from build123d import *

# Parameters (mm, degrees)
F2_SIZE      = 1
F4_DEPTH     = 0.5
F5_T4_DEPTH  = 4.9533840607
F5_T10_DEPTH = 4.9533840607
F5_T16_DEPTH = 4.9533840607
F5_T22_DEPTH = 4.9533840607
F7_DEPTH     = 0.5
F8_T4_DEPTH  = 4.9533840607
F8_T10_DEPTH = 4.9533840607
F8_T16_DEPTH = 4.9533840607
F8_T22_DEPTH = 4.9533840607
F8_T28_DEPTH = 4.9533840607
F8_T34_DEPTH = 4.9533840607
F8_T40_DEPTH = 4.9533840607
F8_T46_DEPTH = 4.9533840607


# Not quite as in the source:
# - a fillet or chamfer that OpenCascade refuses, or shapes differently, is made with other operations: its cross-section is extruded or revolved along the edge and cut away or added


with BuildPart() as f1:
    # F0 (on Right) → F1 (revolve)
    with BuildSketch(Plane.YZ):
        with BuildLine():
            Line((0, 2), (0, 0))
            Line((0, 0), (11, 0))
            Line((11, 0), (11, 1))
            Line((11, 1), (1.5, 1))
            Line((1.5, 1), (1.5, 2.5))
            ThreePointArc((1.5, 2.5), (1.3535533906, 2.8535533906), (1, 3))
            ThreePointArc((1, 3), (0.2928932188, 2.7071067812), (0, 2))
        make_face()
    revolve(axis=Axis((0, -4.3078260496, 0), (0, -1, 0)))

    # F2
    f2_edges = [f1.edges().sort_by_distance(p)[0] for p in [
        (0, 11, -1),
    ]]
    chamfer(f2_edges, length=F2_SIZE)

    # F3 (on Right) → F4 (cut, symmetric)
    with BuildSketch(Plane.YZ):
        Polygon((1.5, 0), (0, 1.85), (0, -1.85), align=None)
    extrude(amount=F4_DEPTH, both=True, mode=Mode.SUBTRACT)

    # F5: chamfer of 0.5 on 4 edges, made by hand


with BuildPart() as f5_tool2:
    # F5_s3 → F5_t4 (new body)
    with BuildSketch(Plane(origin=(0, -1.7148497309, -2.1149813348), x_dir=(1, 0, 0), z_dir=(0, 0.6298019584, 0.7767557487))):
        Polygon((0, 1.1651336231), (0.5, 0.6651336231), (0.5, 1.1651336231), align=None)
    extrude(amount=F5_T4_DEPTH)

    split(bisect_by=Plane.XZ, keep=Keep.BOTTOM)

    split(bisect_by=Plane(origin=(0, 0.9050242398, 0.7338034376), x_dir=(1, 0, 0), z_dir=(0, -0.7767557487, -0.6298019584)), keep=Keep.TOP)


with BuildPart() as f1_1:
    add(f1.part)

    # F5_t1: union F5_tool2
    add(f5_tool2.part)


with BuildPart() as f5_tool8:
    # F5_s9 → F5_t10 (new body)
    with BuildSketch(Plane(origin=(0, -1.7148497309, -2.1149813348), x_dir=(1, 0, 0), z_dir=(0, 0.6298019584, 0.7767557487))):
        Polygon((-0.5, 0.6651336231), (0, 1.1651336231), (-0.5, 1.1651336231), align=None)
    extrude(amount=F5_T10_DEPTH)

    split(bisect_by=Plane.XZ, keep=Keep.BOTTOM)

    split(bisect_by=Plane(origin=(0, 0.9050242398, 0.7338034376), x_dir=(1, 0, 0), z_dir=(0, -0.7767557487, -0.6298019584)), keep=Keep.TOP)


with BuildPart() as f1_2:
    add(f1_1.part)

    # F5_t7: union F5_tool8
    add(f5_tool8.part)


with BuildPart() as f5_tool14:
    # F5_s15 → F5_t16 (new body)
    with BuildSketch(Plane(origin=(0, 1.4048012514, -1.73258821), x_dir=(1, 0, 0), z_dir=(0, -0.6298019584, 0.7767557487))):
        Polygon((-0.5, 0.6651336231), (0, 1.1651336231), (-0.5, 1.1651336231), align=None)
    extrude(amount=F5_T16_DEPTH)

    split(bisect_by=Plane.XZ, keep=Keep.BOTTOM)

    split(bisect_by=Plane(origin=(0, 0.9050242398, -0.7338034376), x_dir=(1, 0, 0), z_dir=(0, -0.7767557487, 0.6298019584)), keep=Keep.TOP)


with BuildPart() as f1_3:
    add(f1_2.part)

    # F5_t13: union F5_tool14
    add(f5_tool14.part)


with BuildPart() as f5_tool20:
    # F5_s21 → F5_t22 (new body)
    with BuildSketch(Plane(origin=(0, 1.4048012514, -1.73258821), x_dir=(1, 0, 0), z_dir=(0, -0.6298019584, 0.7767557487))):
        Polygon((0.5, 0.6651336231), (0, 1.1651336231), (0.5, 1.1651336231), align=None)
    extrude(amount=F5_T22_DEPTH)

    split(bisect_by=Plane.XZ, keep=Keep.BOTTOM)

    split(bisect_by=Plane(origin=(0, 0.9050242398, -0.7338034376), x_dir=(1, 0, 0), z_dir=(0, -0.7767557487, 0.6298019584)), keep=Keep.TOP)


with BuildPart() as f1_4:
    add(f1_3.part)

    # F5_t19: union F5_tool20
    add(f5_tool20.part)

    # F6 (on Top) → F7 (cut, symmetric)
    with BuildSketch(Plane.XY):
        Polygon((0, 1.5), (-1.85, 0), (1.85, 0), align=None)
    extrude(amount=F7_DEPTH, both=True, mode=Mode.SUBTRACT)

    # F8: chamfer of 0.5 on 4 edges, made by hand


with BuildPart() as f8_tool2:
    # F8_s3 → F8_t4 (new body)
    with BuildSketch(Plane(origin=(2.1149813348, -1.7148497309, 0), x_dir=(0, 0, 1), z_dir=(-0.7767557487, 0.6298019584, 0))):
        Polygon((0, 1.1651336231), (-0.5, 0.6651336231), (-0.5, 1.1651336231), align=None)
    extrude(amount=F8_T4_DEPTH)

    split(bisect_by=Plane.XZ, keep=Keep.BOTTOM)

    split(bisect_by=Plane(origin=(0.5825668116, 0.4525121199, -0.3669017188), x_dir=(-0.6134375783, 0.7897432099, 0), z_dir=(0.7071067812, 0.5492492572, -0.4453372356)), keep=Keep.TOP)


with BuildPart() as f1_5:
    add(f1_4.part)

    # F8_t1: union F8_tool2
    add(f8_tool2.part)


with BuildPart() as f8_tool8:
    # F8_s9 → F8_t10 (new body)
    with BuildSketch(Plane(origin=(2.1149813348, -1.7148497309, 0), x_dir=(0, 0, 1), z_dir=(-0.7767557487, 0.6298019584, 0))):
        Polygon((0, 1.1651336231), (-0.5, 0.6651336231), (-0.5, 1.1651336231), align=None)
    extrude(amount=F8_T10_DEPTH)

    split(bisect_by=Plane(origin=(-0.5825668116, 0.4525121199, -0.3669017188), x_dir=(-0.6134375783, -0.7897432099, 0), z_dir=(-0.7071067812, 0.5492492572, -0.4453372356)), keep=Keep.TOP)

    split(bisect_by=Plane(origin=(-0.7338034376, 0.9050242398, 0), x_dir=(0, 0, 1), z_dir=(0.6298019584, -0.7767557487, 0)), keep=Keep.TOP)


with BuildPart() as f1_6:
    add(f1_5.part)

    # F8_t7: union F8_tool8
    add(f8_tool8.part)


with BuildPart() as f8_tool14:
    # F8_s15 → F8_t16 (new body)
    with BuildSketch(Plane(origin=(1.73258821, 1.4048012514, 0), x_dir=(0, 0, 1), z_dir=(-0.7767557487, -0.6298019584, 0))):
        Polygon((-0.5, 0.6651336231), (0, 1.1651336231), (-0.5, 1.1651336231), align=None)
    extrude(amount=F8_T16_DEPTH)

    split(bisect_by=Plane(origin=(0.7338034376, 0.9050242398, 0), x_dir=(0, 0, 1), z_dir=(-0.6298019584, -0.7767557487, 0)), keep=Keep.TOP)

    split(bisect_by=Plane(origin=(0.5825668116, 0.4525121199, -0.3669017188), x_dir=(-0.6134375783, 0.7897432099, 0), z_dir=(0.7071067812, 0.5492492572, -0.4453372356)), keep=Keep.TOP)


with BuildPart() as f1_7:
    add(f1_6.part)

    # F8_t13: union F8_tool14
    add(f8_tool14.part)


with BuildPart() as f8_tool20:
    # F8_s21 → F8_t22 (new body)
    with BuildSketch(Plane(origin=(1.73258821, 1.4048012514, 0), x_dir=(0, 0, 1), z_dir=(-0.7767557487, -0.6298019584, 0))):
        Polygon((-0.5, 0.6651336231), (0, 1.1651336231), (-0.5, 1.1651336231), align=None)
    extrude(amount=F8_T22_DEPTH)

    split(bisect_by=Plane.XZ, keep=Keep.BOTTOM)

    split(bisect_by=Plane(origin=(-0.5825668116, 0.4525121199, -0.3669017188), x_dir=(-0.6134375783, -0.7897432099, 0), z_dir=(-0.7071067812, 0.5492492572, -0.4453372356)), keep=Keep.TOP)


with BuildPart() as f1_8:
    add(f1_7.part)

    # F8_t19: union F8_tool20
    add(f8_tool20.part)


with BuildPart() as f8_tool26:
    # F8_s27 → F8_t28 (new body)
    with BuildSketch(Plane(origin=(2.1149813348, -1.7148497309, 0), x_dir=(0, 0, 1), z_dir=(-0.7767557487, 0.6298019584, 0))):
        Polygon((0, 1.1651336231), (0.5, 0.6651336231), (0.5, 1.1651336231), align=None)
    extrude(amount=F8_T28_DEPTH)

    split(bisect_by=Plane.XZ, keep=Keep.BOTTOM)

    split(bisect_by=Plane(origin=(0.5825668116, 0.4525121199, 0.3669017188), x_dir=(-0.6134375783, 0.7897432099, 0), z_dir=(0.7071067812, 0.5492492572, 0.4453372356)), keep=Keep.TOP)


with BuildPart() as f1_9:
    add(f1_8.part)

    # F8_t25: union F8_tool26
    add(f8_tool26.part)


with BuildPart() as f8_tool32:
    # F8_s33 → F8_t34 (new body)
    with BuildSketch(Plane(origin=(2.1149813348, -1.7148497309, 0), x_dir=(0, 0, 1), z_dir=(-0.7767557487, 0.6298019584, 0))):
        Polygon((0, 1.1651336231), (0.5, 0.6651336231), (0.5, 1.1651336231), align=None)
    extrude(amount=F8_T34_DEPTH)

    split(bisect_by=Plane(origin=(-0.5825668116, 0.4525121199, 0.3669017188), x_dir=(-0.6134375783, -0.7897432099, 0), z_dir=(-0.7071067812, 0.5492492572, 0.4453372356)), keep=Keep.TOP)

    split(bisect_by=Plane(origin=(-0.7338034376, 0.9050242398, 0), x_dir=(0, 0, 1), z_dir=(0.6298019584, -0.7767557487, 0)), keep=Keep.TOP)


with BuildPart() as f1_10:
    add(f1_9.part)

    # F8_t31: union F8_tool32
    add(f8_tool32.part)


with BuildPart() as f8_tool38:
    # F8_s39 → F8_t40 (new body)
    with BuildSketch(Plane(origin=(1.73258821, 1.4048012514, 0), x_dir=(0, 0, 1), z_dir=(-0.7767557487, -0.6298019584, 0))):
        Polygon((0, 1.1651336231), (0.5, 0.6651336231), (0.5, 1.1651336231), align=None)
    extrude(amount=F8_T40_DEPTH)

    split(bisect_by=Plane(origin=(0.5825668116, 0.4525121199, 0.3669017188), x_dir=(-0.6134375783, 0.7897432099, 0), z_dir=(0.7071067812, 0.5492492572, 0.4453372356)), keep=Keep.TOP)

    split(bisect_by=Plane(origin=(0.7338034376, 0.9050242398, 0), x_dir=(0, 0, 1), z_dir=(-0.6298019584, -0.7767557487, 0)), keep=Keep.TOP)


with BuildPart() as f1_11:
    add(f1_10.part)

    # F8_t37: union F8_tool38
    add(f8_tool38.part)


with BuildPart() as f8_tool44:
    # F8_s45 → F8_t46 (new body)
    with BuildSketch(Plane(origin=(1.73258821, 1.4048012514, 0), x_dir=(0, 0, 1), z_dir=(-0.7767557487, -0.6298019584, 0))):
        Polygon((0, 1.1651336231), (0.5, 0.6651336231), (0.5, 1.1651336231), align=None)
    extrude(amount=F8_T46_DEPTH)

    split(bisect_by=Plane.XZ, keep=Keep.BOTTOM)

    split(bisect_by=Plane(origin=(-0.5825668116, 0.4525121199, 0.3669017188), x_dir=(-0.6134375783, -0.7897432099, 0), z_dir=(-0.7071067812, 0.5492492572, 0.4453372356)), keep=Keep.TOP)


with BuildPart() as f1_12:
    add(f1_11.part)

    # F8_t43: union F8_tool44
    add(f8_tool44.part)


solid = f1_12.part
CAD build for the part. Positions are in the model's coordinates, mm. A direction names the side the tool comes from. Give positions to 0.01 mm unless a question says otherwise; leave off trailing zeros. Order: outer loops, then holes, each group sorted by start corner. A loop starts at its lowest first (then second) coordinate and runs counter-clockwise, first axis right, second up. Notation, with made-up numbers: (8, 48.5) - (58, 48.5) arc R26 ccw to (58, 75.5) - close; hole circle Ø6 at (-11.5, 76). An arc over 180 degrees is marked (long way). Answer in a Markdown table with one row per item.
1. Saw through at A-A, the plane y = 4.75. Give the cut face in (x, z).
Data:
| item | result |
|---|---|
| outline | circle Ø2 at (0, 0) |
2. Pull direction Z, two halves, no side cores. Call faces 1 (the conical face through (0, 11, 0)), 2 (the flat face through (1, 1.5, -1)), 3 (the flat face through (0.82, 0.59, -0.19)), 4 (the flat face through (-0.792, 0.612, 0.191)): pulls with the +Z half, pulls with the -Z half, needs draft (parallel to the pull), parting line crosses it, or undercut.
Data:
| item | result |
|---|---|
| face 1 | parting line crosses it |
| face 2 | needs draft |
| face 3 | undercut |
| face 4 | undercut |
3. Tool access for faces 5 (the cylindrical face through (1, 6, 0)), 6 (the flat face through (1, 0, -1)), 7 (the flat face through (0.82, 0.59, 0.19)): list every direction of +Z, -Z, +X, -X, +Y, -Y with a clear straight run to the whole face (end or side of a thin tool).
Data:
| item | result |
|---|---|
| face 5 | +Y |
| face 6 | +Z, -Z, +X, -X, -Y |
| face 7 | -Y |
4. Probe probe 1 along Y at (x, z) = (-0.5, -1.85); probe 2 along Z at (x, y) = (0, 5.75); probe 3 along Y at (x, z) = (1, 2.2). List the from-to ranges inside material, lowest first. Write a range as [from, to].
Data:
| item | result |
|---|---|
| probe 1 | y = [0, 1.5] |
| probe 2 | z = [-1, 1] |
| probe 3 | y = [0.09, 1.5] |
5. Flat gauge pins, fed straight in: pin 1 (1.5 mm diameter, centred on y = 6, z = 1.5, fed in from +X); pin 2 (3 mm diameter, centred on x = -2.5, z = -1.5, fed in from +Y); pin 3 (0.5 mm diameter, centred on y = 0.5, z = -1, fed in from +X). Where does each tip first touch, or does it go through?
Data:
| item | result |
|---|---|
| pin 1 | stops at x = 0.66 |
| pin 2 | stops at y = 1.5 |
| pin 3 | stops at x = 2.83 |
